from build123d import *

# Parameters (mm, degrees)
BOSS_EXTRUDE1_DEPTH  = 100
BOSS_EXTRUDE15_DEPTH = 100
SKETCH12_R           = 10.538298665
CUT_EXTRUDE1_DEPTH   = 100
CUT_EXTRUDE4_DEPTH   = 100


with BuildPart() as part:
    # Sketch1 → Boss-Extrude1 (new body)
    with BuildSketch(Plane(origin=(0, 0, 0), x_dir=(0, 0, -1), z_dir=(1, 0, 0))):
        with BuildLine():
            Line((0, -20.471600717), (30, -20.471600717))
            ThreePointArc((30, -20.471600717), (-5.700994218, 47.06632084), (-78.701931645, 69.578428053))
            Line((-78.701931645, 69.578428053), (-78.701931645, 39.578428053))
            ThreePointArc((-78.701931645, 39.578428053), (-26.914197654, 25.853117404), (0, -20.471600717))
        make_face()
    extrude(amount=BOSS_EXTRUDE1_DEPTH)

    # 3DSketch6 → Boss-Extrude15 (add)
    with BuildSketch(Plane(origin=(100, 39.578428053, 78.701931645), x_dir=(0, 0.7502508437816612, 0.661153288886099), z_dir=(-1, 0, 0))):
        Polygon((0, 0), (10.699765669, -12.141674792), (18.673279749, -21.189706114), (31.636766263, -17.247671387), (88.356194396, 0), (78.117236691, 33.671085949), (35.570814657, 5.010889827), (22.507525313, 19.834598667), align=None)
    extrude(amount=BOSS_EXTRUDE15_DEPTH)

    # Sketch12 → Cut-Extrude1 (cut)
    with BuildSketch(Plane(origin=(0, -11.452264846, 87.90339576), x_dir=(-1, 0, 0), z_dir=(0, 0.12919059900394475, -0.9916197805252788))):
        with Locations(Location((-50, 109.830380232, 0), (0, 0, 90))):
            Circle(SKETCH12_R)
    extrude(amount=-CUT_EXTRUDE1_DEPTH, mode=Mode.SUBTRACT)

    # Sketch13 → Cut-Extrude4 (cut)
    with BuildSketch(Plane(origin=(0, -11.452264846, 87.90339576), x_dir=(-1, 0, 0), z_dir=(0, 0.12919059900394475, -0.9916197805252788))):
        with BuildLine():
            Line((-100, 97.256951485), (-100, 133.014656874))
            Line((-100, 133.014656874), (-100, 156.830890058))
            Line((-100, 156.830890058), (0, 160.198008755))
            Line((0, 160.198008755), (0, 133.014656874))
            Line((0, 133.014656874), (0, 94.208847546))
            ThreePointArc((0, 94.208847546), (-49.07241929, 126.164299771), (-100, 97.256951485))
        make_face()
    extrude(amount=-CUT_EXTRUDE4_DEPTH, mode=Mode.SUBTRACT)


solid = part.part
Geometry check sheet. Reference: the model listing, model coordinates, mm. Coordinates: 2 decimals unless noted, no trailing zeros. Order: outer loops, then holes, each group sorted by start corner. A loop starts at its lowest first (then second) coordinate and runs counter-clockwise, first axis right, second up. Notation, with made-up numbers: M 37,22 L 73,22 A21 cw 73,44 Z; hole C 22,24 d11. An arc over 180 degrees is marked long. Use CSV: the item, a comma, the result in double quotes.
Item 1: Cross-section at A-A on x = 76. Record the cut outline in (y, z).
Returned:
outline,"M -20.47,-30 A99.81 ccw 69.58,78.7 L 69.58,98.46 L 107.77,103.44 L 103.52,136.05 L 39.58,106.95 L 39.58,78.7 A70 cw -20.47,0 Z"
Item 2: Cross-section at D-D on x = 17. Record the cut outline in (y, z), then the cut area to 3 significant figures.
Returned:
outline,"M -20.47,-30 A99.81 ccw 69.58,78.7 L 69.58,98.46 L 102.51,102.75 L 98.47,133.75 L 39.58,106.95 L 39.58,78.7 A70 cw -20.47,0 Z"
area,"5,870 mm2"
Item 3: Cross-section at B-B on y = 73.5. Record the cut outline in (x, z), then the cut area to 3 significant figures.
Returned:
outline,"M 0,98.97 L 100,98.97 L 100,122.39 L 0,122.39 Z"
area,"2,340 mm2"
Item 4: Gauge pin test, flat ends, axial feed: pin 1 Ø13 at (x, z) = (39.5, 86.5) entering from -Y; pin 2 Ø10 at (x, z) = (27.5, 84.5) entering from +Y; pin 3 Ø1.5 at (x, z) = (35, 20.5) entering from +Y; pin 4 Ø12 at (y, z) = (61, 22) entering from -X. Record the tip position at first contact, or that the pin passes through.
Returned:
pin 1,"stops at y = 39.58"
pin 2,"stops at y = 69.58"
pin 3,"stops at y = 57.65"
pin 4,"stops at x = 0"
Item 5: Cross-section at C-C on z = -2. Record the cut outline in (x, y).
Returned:
outline,"M 0,-20.47 L 100,-20.47 L 100,39.97 L 0,39.97 Z"
Item 6: Mould release check, pull along X, two halves, no side actions. Record for faces 1 (the flat face through (51, 69.578, 89)), 2 (the flat face through (100, 36, 41)), 3 (the cylindrical face through (53.165, 105.328, 119.491)): pulls with the +X half, pulls with the -X half, needs draft (parallel to the pull), parting line crosses it, or undercut.
Returned:
face 1,"needs draft"
face 2,"pulls with the +X half"
face 3,"undercut"
Item 7: Thickness scan on line 1 along Y through (x, z) = (13, 96); line 2 along Y through (x, z) = (51.5, 123); line 3 along Z through (x, y) = (49, 56). Record the ranges inside material, lowest first.
Returned:
line 1,"y = 39.58 to 69.58"
line 2,"y = 74.85 to 84.21, 105.25 to 111.23"
line 3,"z = 18.37 to 114.42"
